from build123d import *

# Parameters (mm, degrees)
F0_W     = 60
F0_H     = 30
F1_DEPTH = 30
F2_W     = 28.7048730254
F2_H     = 30
F3_DEPTH = 30
F3_TAPER = 7
F4_R     = 7.3545492497
F5_DEPTH = 30


with BuildPart() as f1:
    # F0 (on Front) → F1 (new body)
    with BuildSketch(Plane.XZ):
        with Locations((-1.2951269746, 1.9989533018)):
            Rectangle(F0_W, F0_H)
    extrude(amount=F1_DEPTH)

    # F2 (on face) → F3 (join)
    with BuildSketch(Plane.XY.offset(16.9989533018)):
        with Locations((14.3524365127, -15)):
            Rectangle(F2_W, F2_H)
    extrude(amount=F3_DEPTH, taper=F3_TAPER)

    # F4 (on face) → F5 (cut)
    with BuildSketch(Plane.XY.offset(46.9989533018)):
        with Locations((14.2463864759, -14.8219969124)):
            Circle(F4_R)
    extrude(amount=-F5_DEPTH, mode=Mode.SUBTRACT)


solid = f1.part
Work out the finished part from the listing and answer in its coordinate system (mm). A direction names the side the tool comes from. Coordinates: 2 decimals unless noted, no trailing zeros. Write each loop counter-clockwise with the first axis right and the second up, starting at its lowest first coordinate (ties: lowest second). Pieces come first, ordered by that corner, then holes. Notation, with made-up numbers: (63, 43) - (111, 43) arc R32 cw to (111, 77) - close; hole circle Ø5 at (17.25, 41.5). An arc over 180 degrees is marked (long way). One line per question, with ' | ' between items.
1) Find section C-C, the plane z = 27. Determine the outline of the cut face in (x, y), and give its area (3 significant figures).
Checks:
outline: (1.23, -28.77) - (27.48, -28.77) - (27.48, -1.23) - (1.23, -1.23) - close; hole circle Ø14.71 at (14.25, -14.82) | area: 553 mm2
2) Find section B-B, the plane x = 10.5. Determine the outline of the cut face in (y, z), and give its area (3 significant figures).
Checks:
outline: (-30, -13) - (0, -13) - (0, 17) - (-3.68, 47) - (-8.49, 47) - (-8.49, 17) - (-21.15, 17) - (-21.15, 47) - (-26.32, 47) - (-30, 17) - close | area: 1,310 mm2
3) Find section A-A, the plane y = -12.25. Determine the outline of the cut face in (x, z), and give its area (3 significant figures).
Checks:
outline: (-31.3, -13) - (28.7, -13) - (28.7, 17) - (25.02, 47) - (21.14, 47) - (21.14, 17) - (7.36, 17) - (7.36, 47) - (3.68, 47) - (0, 17) - (-31.3, 17) - close | area: 2,140 mm2
4) The mould has two halves that part along Y. Classify faces 1 (the face through (8.41, -19.3, 32.21)), 2 (the face through (-2, -30, 2)), 3 (the face through (-2, 0, 2)): +Y half, -Y half, draft (parallel to the pull), parting line (faces both ways), or undercut.
Checks:
face 1: undercut | face 2: -Y half | face 3: +Y half
5) For faces 4 (the face through (-16, -15, 16.999)), 5 (the face through (14, -15, 16.999)), 6 (the face through (14.553, -28.184, 31.789)), determine the directions among +Z, -Z, +X, -X, +Y, -Y from which every point of the face is accessible in a straight line to the end or side of a thin tool.
Checks:
face 4: +Z, -X, +Y, -Y | face 5: +Z | face 6: +Z, +X, -X, -Y
6) Flat-ended cylindrical pins translate along their axes: P1, Ø10, axis at y = -11.5, z = 32, coming from the -X side; P2, Ø4.5, axis at x = 11, y = -13.5, coming from the +Z side. Find the tip coordinate at first contact, or state that the pin passes through.
Checks:
P1: x = 1.23 | P2: z = 17
7) Consider probe 1 along X at (y, z) = (-11.25, 24.5); probe 2 along Z at (x, y) = (-19, -10.75); probe 3 along Y at (x, z) = (7.5, 21). Determine where each line is inside the solid, lowest interval first. Write a range as [from, to].
Checks:
probe 1: [0.92, 7.82], [20.68, 27.78] | probe 2: [-13, 17] | probe 3: [-29.51, -17.75], [-11.89, -0.49]
8) Find section D-D, the plane y = -2. Determine the outline of the cut face in (x, z).
Checks:
outline: (-31.3, -13) - (28.7, -13) - (28.7, 17) - (26.7, 33.29) - (2, 33.29) - (0, 17) - (-31.3, 17) - close
